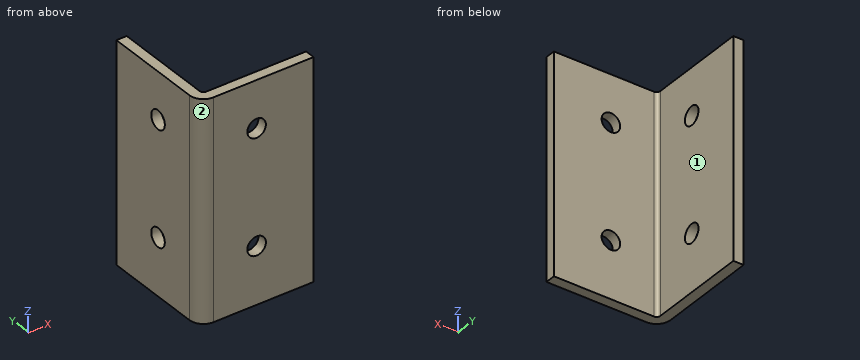
```python
from build123d import *

# Parameters (mm, degrees)
SKETCH1_W                  = 25.4
SKETCH1_H                  = 1498.6
BOSS_EXTRUDE1_DEPTH        = 25.4
SKETCH2_W                  = 23.114
SKETCH2_H                  = 23.114
CUT_EXTRUDE1_DEPTH         = 1499.6
M3_5_CLEARANCE_HOLE1_D     = 4.1402
M3_5_CLEARANCE_HOLE1_DEPTH = 25.4
M3_5_CLEARANCE_HOLE2_D     = 4.1402
M3_5_CLEARANCE_HOLE2_DEPTH = 25.4
CHAMFER1_SIZE              = 2.159
FILLET1_R                  = 0.8128
FILLET2_R                  = 3.0988
SKETCH8_W                  = 95.882963774
SKETCH8_H                  = 79.338329604
CUT_EXTRUDE3_DEPTH         = 1371.6
SKETCH9_W                  = 56.924523055
SKETCH9_H                  = 51.282783217
CUT_EXTRUDE4_DEPTH         = 76.2
SKETCH11_W                 = 51.462522779
SKETCH11_H                 = 66.676735099
CUT_EXTRUDE6_DEPTH         = 2.286


with BuildPart() as part:
    # Sketch1 → Boss-Extrude1 (new body)
    with BuildSketch(Plane(origin=(0, 0, 0), x_dir=(0, -1, 0), z_dir=(-1, 0, 0))):
        with Locations((-12.7, 0)):
            Rectangle(SKETCH1_W, SKETCH1_H)
    extrude(amount=-BOSS_EXTRUDE1_DEPTH)

    # Sketch2 → Cut-Extrude1 (cut, through all)
    with BuildSketch(Plane(origin=(0, 0, -749.3), x_dir=(-1, 0, 0), z_dir=(0, 0, -1))):
        with Locations((-13.843, 13.843)):
            Rectangle(SKETCH2_W, SKETCH2_H)
    extrude(amount=-CUT_EXTRUDE1_DEPTH, mode=Mode.SUBTRACT)

    # M3.5 Clearance Hole1
    with Locations(Plane(origin=(0, 0, 0), x_dir=(-1, 0, 0), z_dir=(0, -1, 0))):
        with Locations((-12.7, 736.6), (-12.7, 711.2), (-12.7, 685.8), (-12.7, 660.4), (-12.7, 635), (-12.7, 609.6), (-12.7, 584.2), (-12.7, 558.8), (-12.7, 533.4), (-12.7, 508), (-12.7, 482.6), (-12.7, 457.2), (-12.7, 431.8), (-12.7, 406.4), (-12.7, 381), (-12.7, 355.6), (-12.7, 330.2), (-12.7, 304.8), (-12.7, 279.4), (-12.7, 254), (-12.7, 228.6), (-12.7, 203.2), (-12.7, 177.8), (-12.7, 152.4), (-12.7, 127), (-12.7, 101.6), (-12.7, 76.2), (-12.7, 50.8), (-12.7, 25.4), (-12.7, 0), (-12.7, -25.4), (-12.7, -50.8), (-12.7, -76.2), (-12.7, -101.6), (-12.7, -127), (-12.7, -152.4), (-12.7, -177.8), (-12.7, -203.2), (-12.7, -228.6), (-12.7, -254), (-12.7, -279.4), (-12.7, -304.8), (-12.7, -330.2), (-12.7, -355.6), (-12.7, -381), (-12.7, -406.4), (-12.7, -431.8), (-12.7, -457.2), (-12.7, -482.6), (-12.7, -508), (-12.7, -533.4), (-12.7, -558.8), (-12.7, -584.2), (-12.7, -609.6), (-12.7, -635), (-12.7, -660.4), (-12.7, -685.8), (-12.7, -711.2), (-12.7, -736.6)):
            Hole(M3_5_CLEARANCE_HOLE1_D / 2, depth=M3_5_CLEARANCE_HOLE1_DEPTH)

    # M3.5 Clearance Hole2
    with Locations(Plane.ZY):
        with Locations((711.2, 12.7), (736.6, 12.7), (685.8, 12.7), (660.4, 12.7), (635, 12.7), (609.6, 12.7), (584.2, 12.7), (558.8, 12.7), (533.4, 12.7), (508, 12.7), (482.6, 12.7), (457.2, 12.7), (431.8, 12.7), (406.4, 12.7), (381, 12.7), (355.6, 12.7), (330.2, 12.7), (304.8, 12.7), (279.4, 12.7), (254, 12.7), (228.6, 12.7), (203.2, 12.7), (177.8, 12.7), (152.4, 12.7), (127, 12.7), (101.6, 12.7), (76.2, 12.7), (50.8, 12.7), (25.4, 12.7), (0, 12.7), (-25.4, 12.7), (-50.8, 12.7), (-76.2, 12.7), (-101.6, 12.7), (-127, 12.7), (-152.4, 12.7), (-177.8, 12.7), (-203.2, 12.7), (-228.6, 12.7), (-254, 12.7), (-279.4, 12.7), (-304.8, 12.7), (-330.2, 12.7), (-355.6, 12.7), (-381, 12.7), (-406.4, 12.7), (-431.8, 12.7), (-457.2, 12.7), (-482.6, 12.7), (-508, 12.7), (-533.4, 12.7), (-558.8, 12.7), (-584.2, 12.7), (-609.6, 12.7), (-635, 12.7), (-660.4, 12.7), (-685.8, 12.7), (-711.2, 12.7), (-736.6, 12.7)):
            Hole(M3_5_CLEARANCE_HOLE2_D / 2, depth=M3_5_CLEARANCE_HOLE2_DEPTH)

    # Chamfer1
    chamfer1_edges = [part.edges().sort_by_distance(p)[0] for p in [
        (25.4, 1.143, -749.3),
        (1.143, 25.4, 749.3),
        (1.143, 25.4, -749.3),
        (25.4, 1.143, 749.3),
    ]]
    chamfer(chamfer1_edges, length=CHAMFER1_SIZE)

    # Fillet1
    fillet1_edges = [part.edges().sort_by_distance(p)[0] for p in [
        (2.286, 2.286, 0),
    ]]
    fillet(fillet1_edges, radius=FILLET1_R)

    # Fillet2
    fillet2_edges = [part.edges().sort_by_distance(p)[0] for p in [
        (0, 0, 0),
    ]]
    fillet(fillet2_edges, radius=FILLET2_R)

    # Sketch8 → Cut-Extrude3 (cut)
    with BuildSketch(Plane.XY.offset(749.3)):
        with Locations((2.286, 3.0988)):
            Rectangle(SKETCH8_W, SKETCH8_H)
    extrude(amount=-CUT_EXTRUDE3_DEPTH, mode=Mode.SUBTRACT)

    # Sketch9 → Cut-Extrude4 (cut)
    with BuildSketch(Plane(origin=(0, 0, -749.3), x_dir=(-1, 0, 0), z_dir=(0, 0, -1))):
        with Locations((-2.180776643, 1.30746368)):
            Rectangle(SKETCH9_W, SKETCH9_H)
    extrude(amount=-CUT_EXTRUDE4_DEPTH, mode=Mode.SUBTRACT)

    # Sketch11 → Cut-Extrude6 (cut)
    with BuildSketch(Plane.XY.offset(-622.3)):
        with Locations((1.85517497, 1.74884985)):
            Rectangle(SKETCH11_W, SKETCH11_H)
    extrude(amount=-CUT_EXTRUDE6_DEPTH, mode=Mode.SUBTRACT)


solid = part.part
```
The model under review builds one solid part; all positions refer to its coordinate system, in mm. Face numbers are marked on the shaded views. A direction names the side the tool comes from. Give positions to 0.01 mm unless a question says otherwise; leave off trailing zeros. Write each loop counter-clockwise with the first axis right and the second up, starting at its lowest first coordinate (ties: lowest second). Pieces come first, ordered by that corner, then holes. Notation, with made-up numbers: M -15.75,81 L 28.25,81 A22 ccw 28.25,99 Z; hole C 49.25,44 d11. An arc over 180 degrees is marked long. Answer in a Markdown table with one row per item.
Item 1: Add section B-B on y = 12.7. Give the boundary of the cut face in (x, z).
Check sheet entries:
| item | result |
|---|---|
| outline | M 0,-673.1 L 2.29,-673.1 L 2.29,-662.47 L 0,-662.47 Z; M 0,-658.33 L 2.29,-658.33 L 2.29,-637.07 L 0,-637.07 Z; M 0,-632.93 L 2.29,-632.93 L 2.29,-624.59 L 0,-624.59 Z |
Item 2: For P1, Ø8, axis at y = 6.5, z = -645, coming from the +X side; P2, Ø5, axis at y = 6.5, z = -635.5, coming from the +X side; P3, Ø5, axis at x = 10, z = -635, coming from the +Y side; P4, Ø2.5, axis at y = 12.7, z = -660.4, coming from the +X side, all flat-tipped, find the tip position at first contact; note any pin that passes through.
Check sheet entries:
| item | result |
|---|---|
| P1 | x = 2.55 |
| P2 | x = 2.29 |
| P3 | y = 2.29 |
| P4 | through |
Item 3: For line 1 along Z through (x, y) = (12.7, 0.9); line 2 along X through (y, z) = (3.5, -667.5), list the stretches that pass through material, from the lowest coordinate up.
Check sheet entries:
| item | result |
|---|---|
| line 1 | -673.1 to -662.47, -658.33 to -637.07, -632.93 to -624.59 |
| line 2 | 0 to 2.29 |
Item 4: Add section A-A on z = -635. Give the boundary of the cut face in (x, y), plus the area to 3 significant figures.
Check sheet entries:
| item | result |
|---|---|
| outline | M 0,3.1 A3.1 ccw 3.1,0 L 10.63,0 L 10.63,2.29 L 3.1,2.29 A0.81 cw 2.29,3.1 L 2.29,10.63 L 0,10.63 Z; M 0,14.77 L 2.29,14.77 L 2.29,25.4 L 0,25.4 Z; M 14.77,0 L 25.4,0 L 25.4,2.29 L 14.77,2.29 Z |
| area | 90.1 mm2 |
Item 5: Tool access review of the marked faces 1 and 2: name each direction out of +Z, -Z, +X, -X, +Y, -Y from which nothing blocks a thin tool from reaching the whole face with its end or side.
Check sheet entries:
| item | result |
|---|---|
| face 1 | +Z, -Z, +X, +Y |
| face 2 | +Z, -Z, -X, -Y |
Item 6: Add section D-D on z = -652.5. Give the boundary of the cut face in (x, y).
Check sheet entries:
| item | result |
|---|---|
| outline | M 0,3.1 A3.1 ccw 3.1,0 L 25.4,0 L 25.4,2.29 L 3.1,2.29 A0.81 cw 2.29,3.1 L 2.29,25.4 L 0,25.4 Z |
